Here's the drawing with two shaded views (mm, measured from the low corner). I have some questions. Give positions to 0.01 mm unless a question says otherwise; leave off trailing zeros. Order: outer loops, then holes, each group sorted by start corner. A loop starts at its lowest first (then second) coordinate and runs counter-clockwise, first axis right, second up. Notation, with made-up numbers: M -23.75,4.5 L 32.25,4.5 A18 ccw 32.25,17.5 Z; hole C 89,84.25 d11. An arc over 180 degrees is marked long. Write each question's results on one line, items separated by ' | '.
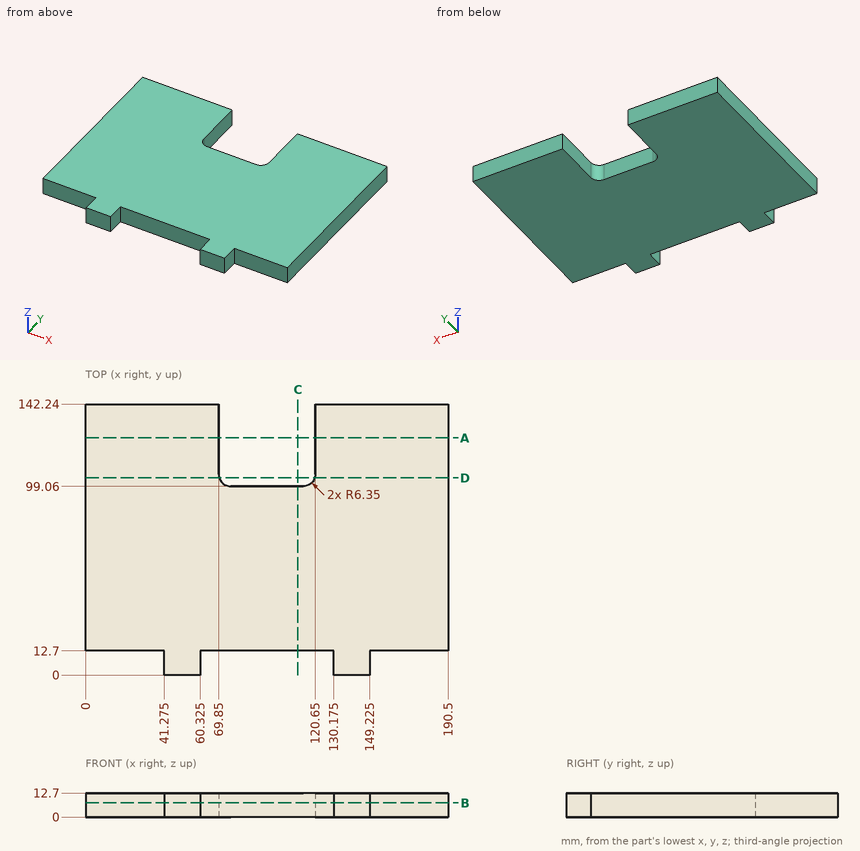
(1) Imagine slicing it at C-C, the plane x = 111.5. Write out the boundary of the cut face in (y, z), plus the area to 3 significant figures.
Data:
outline: M 12.7,0 L 99.06,0 L 99.06,12.7 L 12.7,12.7 Z | area: 1,100 mm2
(2) Imagine slicing it at A-A, the plane y = 124.5. Write out the boundary of the cut face in (x, z), plus the area to 3 significant figures.
Data:
outline: M 0,0 L 69.85,0 L 69.85,12.7 L 0,12.7 Z; M 120.65,0 L 190.5,0 L 190.5,12.7 L 120.65,12.7 Z | area: 1,770 mm2
(3) I need wall thicknesses on L1, parallel to X at y = 6.5, z = 3.5 (3 decimals); L2, parallel to X at y = 115.5, z = 7.25; L3, parallel to Y at x = 109, z = 2.25. Which ranges of each line are inside material? Lowest first, please. Write a range as from..to.
Data:
L1: x = 41.275..60.325, 130.175..149.225 | L2: x = 0..69.85, 120.65..190.5 | L3: y = 12.7..99.06
(4) Will these pins go through, and if not, where does the flat tip stop? P1, Ø1, axis at x = 171, y = 124.5, coming from the -Z side; P2, Ø4, axis at y = 4.5, z = 6, coming from the -X side (3 decimals); P3, Ø5, axis at x = 107, z = 1.5, coming from the +Y side; P4, Ø6.5, axis at y = 6.5, z = 8, coming from the +X side (3 decimals).
Data:
P1: stops at z = 0 | P2: stops at x = 41.275 | P3: stops at y = 99.06 | P4: stops at x = 149.225
(5) Imagine slicing it at D-D, the plane y = 103.5. Write out the boundary of the cut face in (x, z).
Data:
outline: M 0,0 L 70.14,0 L 70.14,12.7 L 0,12.7 Z; M 120.36,0 L 190.5,0 L 190.5,12.7 L 120.36,12.7 Z
(6) Imagine slicing it at B-B, the plane z = 7.5. Write out the boundary of the cut face in (x, y) (3 decimals), plus the area to 3 significant figures.
Data:
outline: M 0,12.7 L 41.275,12.7 L 41.275,0 L 60.325,0 L 60.325,12.7 L 130.175,12.7 L 130.175,0 L 149.225,0 L 149.225,12.7 L 190.5,12.7 L 190.5,142.24 L 120.65,142.24 L 120.65,105.41 A6.35 cw 114.3,99.06 L 76.2,99.06 A6.35 cw 69.85,105.41 L 69.85,142.24 L 0,142.24 Z | area: 23,000 mm2
